Geometry check sheet. Reference: the model listing, model coordinates, mm. A direction names the side the tool comes from. Give positions to 0.01 mm unless a question says otherwise; leave off trailing zeros. Write each loop counter-clockwise with the first axis right and the second up, starting at its lowest first coordinate (ties: lowest second). Pieces come first, ordered by that corner, then holes. Notation, with made-up numbers: (-4, 70.25) - (29, 70.25) arc R9 ccw to (29, 87.25) - close; hole circle Ø3 at (41.5, 75). An arc over 180 degrees is marked (long way). One line per question, with ' | ' between items. Start each with the question number.
Q1. Section check B-B on x = -8. Record the boundary of the cut face in (y, z), and give its area (3 significant figures).
Q2. Section check C-C on z = -13.5. Record the boundary of the cut face in (x, y).
Q3. Set-up check for faces 5 (the face through (85, -3, -1.67)), 6 (the face through (71.425, 1.014, 15.539)), 7 (the face through (-56, -4, -31.563)): record each of +Z, -Z, +X, -X, +Y, -Y from which the full face is reachable in a straight line by a thin tool's end or side.
Q4. Thickness scan on L1, parallel to X at y = -6.75, z = -2; L2, parallel to X at y = 0.25, z = -16; L3, parallel to Y at x = 62.5, z = 38.5. Record the ranges inside material, lowest first. Write a range as [from, to].
Q5. Gauge pin test, flat ends, axial feed: P1, Ø0.5, axis at y = 0.5, z = -34.5, coming from the -X side; P2, Ø0.6, axis at y = 0.5, z = -25, coming from the -X side; P3, Ø1.5, axis at x = 85, y = -1, coming from the +Z side. Record the tip position at first contact, or that the pin passes through.
Q6. Section check A-A on y = -3.5. Record the boundary of the cut face in (x, z).
Q7. Release check for a two-part mould opening along Z. For faces 1 (the face through (35, 0, -31)), 2 (the face through (78.69, 1.01, 19.58)), 3 (the face through (71.6, 1, -20.2)), 4 (the face through (85, -3, -3.67)) record: +Z half, -Z half, draft (parallel to the pull), parting line (faces both ways), or undercut.
```python
from build123d import *

# Parameters (mm, degrees)
BOSS_EXTRUDE1_DEPTH = 2
EDGE_FLANGE1_DEPTH  = 2
EDGE_FLANGE2_DEPTH  = 2
CUT_EXTRUDE3_DEPTH  = 10


# Sheet-metal steps are written as plain solids
with BuildPart() as part:
    # Sketch2 → Boss-Extrude1 (new body)
    with BuildSketch(Plane(origin=(0, 0, 0), x_dir=(1, 0, 0), z_dir=(0, 1, 0))):
        Polygon((81.609993248, 1.669814581), (81.609993248, -16.836643227), (75.909994488, -22.536641987), (75.909994488, -38.936642207), (70.009993588, -44.836643107), (58.109994528, -44.836643107), (58.109994528, -34.336641247), (63.809993288, -34.336641247), (67.509993508, -30.636641027), (67.509993508, -19.345596807), (75.109993548, -11.745596767), (75.109993548, 16.463358753), (67.709993108, 23.863356653), (67.709993108, 26.763358473), (64.309994828, 30.163356753), (-43.190006072, 30.163356753), (-52.793309772, 30.163356753), (-52.793309772, 31.563357033), (-54.793309772, 31.563357033), (-54.793309772, 33.563357033), (-52.793309772, 33.563357033), (-52.793309772, 34.963357313), (-43.190006072, 34.963357313), (66.209993568, 34.963357313), (81.609993248, 19.563357633), (81.609993248, 3.669814581), (83.609993248, 3.669814581), (83.609993248, 1.669814581), align=None)
    extrude(amount=BOSS_EXTRUDE1_DEPTH)

    # Edge-Flange1 section (across the edge) → Edge-Flange1 (add)
    with BuildSketch(Plane(origin=(-55.793309772, 0, -31.563357033), x_dir=(1, 0, 0), z_dir=(0, 0, -1))):
        with BuildLine():
            Line((-2, 0.5), (-2, 10))
            Line((-2, 10), (0, 10))
            Line((0, 10), (0, 0.5))
            ThreePointArc((0, 0.5), (0.146446609, 0.146446609), (0.5, 0))
            Line((0.5, 0), (1, 0))
            Line((1, 0), (1, -2))
            Line((1, -2), (0.5, -2))
            ThreePointArc((0.5, -2), (-1.267766953, -1.267766953), (-2, 0.5))
        make_face()
    extrude(amount=EDGE_FLANGE1_DEPTH)

    # Edge-Flange2 section (across the edge) → Edge-Flange2 (add)
    with BuildSketch(Plane(origin=(84.609993248, 0, -3.669814581), x_dir=(-1, 0, 0), z_dir=(0, 0, 1))):
        with BuildLine():
            Line((-2, 0.5), (-2, 10))
            Line((-2, 10), (0, 10))
            Line((0, 10), (0, 0.5))
            ThreePointArc((0, 0.5), (0.146446609, 0.146446609), (0.5, 0))
            Line((0.5, 0), (1, 0))
            Line((1, 0), (1, -2))
            Line((1, -2), (0.5, -2))
            ThreePointArc((0.5, -2), (-1.267766953, -1.267766953), (-2, 0.5))
        make_face()
    extrude(amount=EDGE_FLANGE2_DEPTH)

    # Sketch13 → Cut-Extrude3 (cut)
    with BuildSketch(Plane(origin=(0, 2, 0), x_dir=(1, 0, 0), z_dir=(0, 1, 0))):
        Polygon((64.364993832, 30.231358373), (-43.077006168, 30.231358373), (-52.793309772, 30.231358373), (-52.793309772, 30.163356753), (64.309994828, 30.163356753), (67.709993108, 26.763358473), (67.709993108, 23.863356653), (75.109993548, 16.463358753), (75.109993548, -11.745596767), (67.509993508, -19.345596807), (67.509993508, -30.636641027), (63.809993288, -34.336641247), (58.109994528, -34.336641247), (58.109994528, -44.836643107), (70.009993588, -44.836643107), (75.909994488, -38.936642207), (75.909994488, -22.536641987), (81.609993248, -16.836643227), (81.609993248, 1.669814581), (81.509993832, 1.669814581), (81.509993832, -16.758641627), (75.794993832, -22.473641627), (75.794993832, -38.856641627), (71.222993832, -43.428641627), (58.268993832, -43.428641627), (58.268993832, -35.554641627), (65.126993832, -35.554641627), (67.665284412, -33.016351047), (67.669899592, -19.298575587), (75.286993832, -11.672504987), (75.286993832, 16.515358373), (67.793993832, 24.008355833), (67.793993832, 26.802358373), align=None)
        Polygon((-52.793309772, 30.163356753), (-52.793309772, 30.231358373), (-53.09278865, 30.231358373), (-53.09278865, 29.122247983), (64.073173088, 29.122247983), (66.904295046, 26.802358373), (66.904295046, 23.685270997), (74.890508664, 15.670381273), (73.855495628, -9.951608799), (66.571415804, -17.811521066), (66.392045366, -24.291741654), (65.126993832, -32.125935595), (57.650093481, -33.249786732), (57.276841603, -46.73447534), (58.268993832, -46.73447534), (69.513593476, -46.73447534), (76.944541222, -41.148796497), (77.641700893, -23.890445583), (84.109993248, -17.212504202), (84.109993248, 1.669814581), (81.609993248, 1.669814581), (81.609993248, -16.836643227), (75.909994488, -22.536641987), (75.909994488, -38.936642207), (70.009993588, -44.836643107), (58.109994528, -44.836643107), (58.109994528, -34.336641247), (63.809993288, -34.336641247), (67.509993508, -30.636641027), (67.509993508, -19.345596807), (75.109993548, -11.745596767), (75.109993548, 16.463358753), (67.709993108, 23.863356653), (67.709993108, 26.763358473), (64.309994828, 30.163356753), align=None)
        Polygon((84.109993248, 19.032357692), (84.109993248, 3.669814581), (81.509993832, 3.669814581), (81.509993832, 19.436358373), (66.015993832, 34.930358373), (62.967993832, 34.930358373), (62.967993832, 33.914358373), (60.681993832, 33.914358373), (60.681993832, 34.930358373), (48.489993832, 34.930358373), (48.489993832, 33.914358373), (46.203993832, 33.914358373), (46.203993832, 34.930358373), (33.376993832, 34.930358373), (33.376993832, 33.914358373), (30.963993832, 33.914358373), (30.963993832, 34.930358373), (18.644993832, 34.930358373), (18.644993832, 33.914358373), (16.358993832, 33.914358373), (16.358993832, 34.930358373), (3.912993832, 34.930358373), (3.912993832, 33.914358373), (1.499993832, 33.914358373), (1.499993832, 34.930358373), (-11.327006168, 34.930358373), (-11.327006168, 33.914358373), (-13.740006168, 33.914358373), (-13.740006168, 34.930358373), (-26.567006168, 34.930358373), (-26.567006168, 33.914358373), (-28.980006168, 33.914358373), (-28.980006168, 34.930358373), (-41.172006168, 34.930358373), (-41.172006168, 33.914358373), (-44.172006168, 33.914358373), (-44.172006168, 34.930358373), (-54.307784522, 34.930358373), (-54.307784522, 35.697895733), (66.904295046, 35.697895733), align=None)
    extrude(amount=-CUT_EXTRUDE3_DEPTH, mode=Mode.SUBTRACT)


solid = part.part
```
Working result:
1) outline: (0, -34.93) - (2, -34.93) - (2, -30.23) - (0, -30.23) - close | area: 9.40 mm2
2) outline: (75.29, 0) - (81.51, 0) - (81.51, 2) - (75.29, 2) - close
3) face 5: +Z, +X, +Y, -Y | face 6: -X, +Y, -Y | face 7: +Z, -X, +Y, -Y
4) L1: x = [84.61, 86.61] | L2: x = [75.29, 81.51] | L3: y = [0, 2]
5) P1: stops at x = -52.79 | P2: stops at x = 67.79 | P3: stops at z = -1.67
6) outline: (-57.79, -33.56) - (-55.79, -33.56) - (-55.79, -31.56) - (-57.79, -31.56) - close; (84.61, -3.67) - (86.61, -3.67) - (86.61, -1.67) - (84.61, -1.67) - close
7) face 1: draft | face 2: +Z half | face 3: undercut | face 4: -Z half
